```python
from build123d import *

# Parameters (mm, degrees)
F0_R      = 64
F1_DEPTH  = 25.5
F2_R      = 58
F3_DEPTH  = 1
F4_SIZE   = 8
F5_R      = 30
F6_DEPTH  = 6
F7_SIZE   = 5.99999
F9_R      = 9
F10_DEPTH = 18


# Not quite as in the source:
# - a fillet or chamfer is up to 0.001 mm smaller than in the source, because OpenCascade refuses the exact size


with BuildPart() as f1:
    # F0 (on Front) → F1 (new body)
    with BuildSketch(Plane.XZ):
        Circle(F0_R)
    extrude(amount=F1_DEPTH)

    # F2 (on face) → F3 (cut)
    with BuildSketch(Plane(origin=(0, 0, 0), x_dir=(-1, 0, 0), z_dir=(0, 1, 0))):
        Circle(F2_R)
    extrude(amount=-F3_DEPTH, mode=Mode.SUBTRACT)

    # F4
    f4_edges = [f1.edges().sort_by_distance(p)[0] for p in [
        (-64, -25.5, 0),
    ]]
    chamfer(f4_edges, length=F4_SIZE)

    # F5 (on face) → F6 (join)
    with BuildSketch(Plane.XZ.offset(25.5)):
        Circle(F5_R)
    extrude(amount=F6_DEPTH)

    # F7 (size 6 in the source; OpenCascade refuses exactly that, so slightly less here)
    f7_edges = [f1.edges().sort_by_distance(p)[0] for p in [
        (-30, -31.5, 0),
    ]]
    chamfer(f7_edges, length=F7_SIZE)

    # F9 (on face) → F10 (cut)
    with BuildSketch(Plane.XZ.offset(31.5)):
        Circle(F9_R)
    extrude(amount=-F10_DEPTH, mode=Mode.SUBTRACT)


solid = f1.part
```
Verification items for the finished model (mm, model axes). A direction names the side the tool comes from. Coordinates: 2 decimals unless noted, no trailing zeros. Loops run counter-clockwise (first coordinate to the right, second up) from the corner with the lowest first, then second, coordinate; pieces in that order, holes last. Notation, with made-up numbers: (21.25, -19) -> (40.25, -19) arc R34 cw to (40.25, 13) -> close; hole circle Ø1 at (56, 57). An arc over 180 degrees is marked (long way). Answer in a Markdown table with one row per item. Add a question column.
1. Draft check along X on faces 1 (the face through (-24.268, -31.209, 1.068)), 2 (the face through (10, -31.5, 0)), 3 (the face through (0, -13.5, 0)). Enter one of: +X half, -X half, draft (parallel to the pull), parting line (faces both ways), or undercut.
2. Access from +Z, -Z, +X, -X, +Y, -Y to the whole of each face (thin tool, end or side, straight path). Record for faces 4 (the face through (-13.87, -8.63, -62.48)), 5 (the face through (1, -1, 1)), 6 (the face through (-1.172, -22.626, 8.923)).
3. Section check C-C, the plane y = -27. Enter the section's corners in (x, z).
4. Material ranges on probe 1 along Z at (x, y) = (0, -23.5); probe 2 along Z at (x, y) = (0, -0.6); probe 3 along Y at (x, z) = (51, -22), recorded low to high. Write a range as [from, to].
5. Section check D-D, the plane y = -15.5. Enter the section's corners in (x, z).
6. Depth check by flat-ended pin: P1, Ø5, axis at y = -6, z = 5, coming from the +X side; P2, Ø4, axis at x = 22, z = 13, coming from the +Y side; P3, Ø8, axis at y = -9, z = -28.5, coming from the -X side. Enter the tip coordinate at first touch or a pass-through.
Derived:
| question | item | result |
|---|---|---|
| 1 | face 1 | parting line |
| 1 | face 2 | draft |
| 1 | face 3 | undercut |
| 2 | face 4 | +Y, -Y |
| 2 | face 5 | +Y |
| 2 | face 6 | -Y |
| 3 | outline | circle Ø57 at (0, 0); hole circle Ø18 at (0, 0) |
| 4 | probe 1 | z = [-58, -9], [9, 58] |
| 4 | probe 2 | z = [-64, -58], [58, 64] |
| 4 | probe 3 | y = [-25.5, -1] |
| 5 | outline | circle Ø128 at (0, 0); hole circle Ø18 at (0, 0) |
| 6 | P1 | stops at x = 63.95 |
| 6 | P2 | stops at y = -1 |
| 6 | P3 | stops at x = -59.12 |
